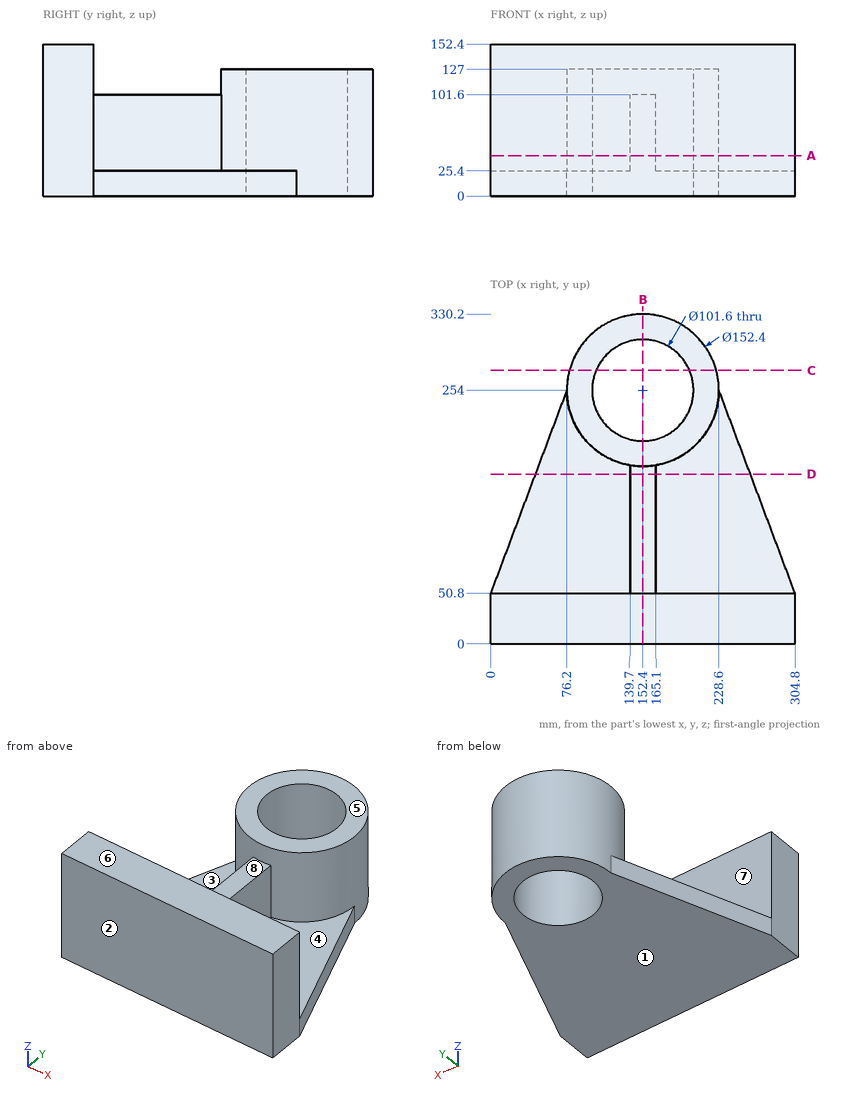
Geometry: see drawing. Coordinates: mm, zero at the bounding-box minimum. A direction names the side the tool comes from. Give positions to 0.01 mm unless a question says otherwise; leave off trailing zeros. Order: outer loops, then holes, each group sorted by start corner. A loop starts at its lowest first (then second) coordinate and runs counter-clockwise, first axis right, second up. Notation, with made-up numbers: (-11.5, 11.5) -> (17.5, 11.5) arc R29 cw to (17.5, 37.5) -> close; hole circle Ø4 at (1.5, 6). An arc over 180 degrees is marked (long way). Write each question's results on one line, items separated by ' | '. Start each with the question number.
1) Section A-A (z = 40.5). Return loops of the section in (x, y).
2) Section C-C (y = 274). Return loops of the section in (x, z).
3) First-contact query: pin 1 (23 mm diameter, centred on y = 125.5, z = 47.5, fed in from +X); pin 2 (6 mm diameter, centred on x = 84, y = 223.5, fed in from -Z); pin 3 (3 mm diameter, centred on y = 74.5, z = 23.5, fed in from +X) (3 decimals); pin 4 (12 mm diameter, centred on x = 195, y = 62, fed in from +Z). Flat tips, straight axial feed; report the tip coordinate or a pass-through.
4) Section B-B (x = 152.4). Return loops of the section in (y, z).
5) Draft query along Y for the marked faces 1, 2 and 3. Return one class per face: pulls with the +Y half, pulls with the -Y half, needs draft (parallel to the pull), parting line crosses it, or undercut.
6) Section D-D (y = 170). Return loops of the section in (x, z).
7) Line query: line 1 (Y direction, x = 117.5, z = 124); line 2 (Y direction, x = 157, z = 105); line 3 (Y direction, x = 152, z = 58). Output: solid intervals per line, ascending. Write a range as from..to.
8) Set-up query: the marked faces 4, 5, 6, 7 and 8. Return all of +Z, -Z, +X, -X, +Y, -Y with unobstructed straight access to the full face (end or side cutting, diameter ignored); none if empty.
Calculated:
1) outline: (0, 0) -> (304.8, 0) -> (304.8, 50.8) -> (165.1, 50.8) -> (165.1, 178.87) arc R76.2 ccw (long way) to (139.7, 178.87) -> (139.7, 50.8) -> (0, 50.8) -> close; hole circle Ø101.6 at (152.4, 254)
2) outline: (78.87, 0) -> (105.7, 0) -> (105.7, 127) -> (78.87, 127) -> close; (199.1, 0) -> (225.93, 0) -> (225.93, 127) -> (199.1, 127) -> close
3) pin 1: x = 165.1 | pin 2: z = 0 | pin 3: x = 296.475 | pin 4: z = 25.4
4) outline: (0, 0) -> (203.2, 0) -> (203.2, 127) -> (177.8, 127) -> (177.8, 101.6) -> (50.8, 101.6) -> (50.8, 152.4) -> (0, 152.4) -> close; (304.8, 0) -> (330.2, 0) -> (330.2, 127) -> (304.8, 127) -> close
5) face 1: needs draft | face 2: pulls with the -Y half | face 3: undercut
6) outline: (44.7, 0) -> (260.1, 0) -> (260.1, 25.4) -> (165.1, 25.4) -> (165.1, 101.6) -> (139.7, 101.6) -> (139.7, 25.4) -> (44.7, 25.4) -> close
7) line 1: 0..50.8, 186.26..217.09, 290.91..321.74 | line 2: 0..50.8, 177.94..203.41, 304.59..330.06 | line 3: 0..203.2, 304.8..330.2
8) face 4: +Z, +X | face 5: +Z, +X, -X, +Y | face 6: +Z, +X, -X, +Y, -Y | face 7: +Z | face 8: +Z, +X, -X
